from build123d import *

# Parameters (mm, degrees)
F1_DEPTH = 500
F2_DEPTH = 400
F3_T     = -22
F5_DEPTH = 25


# Not quite as in the source:
# - a shell that OpenCascade refuses in one call is made with other operations: the cavity is built on its own and cut out


with BuildPart() as f1:
    # F0 (on Top) → F1 (new body)
    with BuildSketch(Plane.XY):
        Polygon((0, 0), (-1050, 0), (-1050, -22), (-420.8932188135, -22), (-22, -420.8932188135), (-22, -1028), (-500, -1028), (-500, -1050), (0, -1050), align=None)
        Polygon((-389.7805204412, -22), (-22, -22), (-22, -389.7805204412), align=None, mode=Mode.SUBTRACT)
        Polygon((-420.8932188135, -22), (-1050, -22), (-1050, -500), (-650, -500), (-500, -650), (-500, -1028), (-22, -1028), (-22, -420.8932188135), align=None)
    extrude(amount=-F1_DEPTH)

    # F0 (on Top) → F2 (join)
    with BuildSketch(Plane.XY):
        Polygon((0, 0), (-1050, 0), (-1050, -22), (-420.8932188135, -22), (-22, -420.8932188135), (-22, -1028), (-500, -1028), (-500, -1050), (0, -1050), align=None)
        Polygon((-389.7805204412, -22), (-22, -22), (-22, -389.7805204412), align=None, mode=Mode.SUBTRACT)
    extrude(amount=F2_DEPTH)

    # F3: a shell. OpenCascade refuses it in one call, so the cavity is built on its own and cut out:
    # the body offset inwards by the wall thickness, plus a prism from it out through each open face.
    f3_core = offset(f1.part, amount=F3_T, kind=Kind.INTERSECTION, mode=Mode.PRIVATE)
    f3_exits = [f3_core.faces().sort_by_distance(p)[0] for p in [
        (-463.695201, -463.695201, -478),
    ]]
    add(f3_core, mode=Mode.SUBTRACT)
    extrude(f3_exits, amount=-F3_T, mode=Mode.SUBTRACT)

    # F4 (on face) → F5 (cut)
    with BuildSketch(Plane.XZ.offset(1050)):
        with BuildLine():
            ThreePointArc((-500, 248), (-455.4802307404, 355.4802307404), (-348, 400))
            Line((-348, 400), (-500, 400))
            Line((-500, 400), (-500, 248))
        make_face()
    extrude(amount=-F5_DEPTH, mode=Mode.SUBTRACT)


solid = f1.part
Build history of the part. All positions in model axes, mm. A direction names the side the tool comes from. Coordinates: 2 decimals unless noted, no trailing zeros. Order: outer loops, then holes, each group sorted by start corner. A loop starts at its lowest first (then second) coordinate and runs counter-clockwise, first axis right, second up. Notation, with made-up numbers: (55, 14.5) - (95, 14.5) arc R17 cw to (95, 33.5) - close; hole circle Ø8 at (87.5, 6). An arc over 180 degrees is marked (long way). Write each question's results on one line, items separated by ' | '. Start each with the question number.
Item 1: Band-saw the part on A-A on z = -104.5. Write the cut outline in (x, y), and give its area (3 significant figures).
Item 2: Mould opens along X. For faces 1 (the face through (0, -532, -56)), 2 (the face through (-500, -847, -214)), 3 (the face through (-560.584, -558.303, -257.654)), 4 (the face through (-740, -22, 197)) say: released by +X, released by -X, zero draft, split by the parting line, or undercut.
Item 3: Wall check: probe 1 along X at (y, z) = (-684, -312.5); probe 2 along X at (y, z) = (-324, -179). Give the ranges that are in metal, low to high. Write a range as [from, to].
Item 4: Band-saw the part on C-C on y = -343. Write the cut outline in (x, z).
Item 5: Band-saw the part on B-B on x = -149.5. Write the cut outline in (y, z), and give its area (3 significant figures).
Item 6: Band-saw the part on D-D on z = 288. Write the cut outline in (x, y).
Item 7: Flat gauge pins, fed straight in: pin 1 (4 mm diameter, centred on y = -740.5, z = 138, fed in from -X); pin 2 (5 mm diameter, centred on x = -633.5, y = -131.5, fed in from -Z). Where does each tip first touch, or does it go through?
Item 8: Tool access for faces 5 (the face through (-203.32, -208.46, -56.3)), 6 (the face through (-429, -406, 0)), 7 (the face through (-247, -1028, -258)), 8 (the face through (-853, -500, -246)): list every direction of +Z, -Z, +X, -X, +Y, -Y with a clear straight run to the whole face (end or side of a thin tool).
Numbers:
1) outline: (-1050, -500) - (-650, -500) - (-500, -650) - (-500, -1050) - (0, -1050) - (0, 0) - (-1050, 0) - close; hole (-1028, -478) - (-640.89, -478) - (-478, -640.89) - (-478, -1028) - (-22, -1028) - (-22, -420.89) - (-420.89, -22) - (-1028, -22) - close; hole (-389.78, -22) - (-22, -389.78) - (-22, -22) - close | area: 100,000 mm^2
2) face 1: released by +X | face 2: released by -X | face 3: undercut | face 4: zero draft
3) probe 1: [-500, -478], [-22, 0] | probe 2: [-1050, -1028], [-118.89, -87.78], [-22, 0]
4) outline: (-1050, -500) - (-1028, -500) - (-1028, -22) - (-99.89, -22) - (-99.89, -500) - (-68.78, -500) - (-68.78, 400) - (-99.89, 400) - (-99.89, 0) - (-1050, 0) - close; (-22, -500) - (0, -500) - (0, 400) - (-22, 400) - close
5) outline: (-1050, -500) - (-1028, -500) - (-1028, -22) - (-293.39, -22) - (-293.39, -500) - (-262.28, -500) - (-262.28, 400) - (-293.39, 400) - (-293.39, 0) - (-1028, 0) - (-1028, 400) - (-1050, 400) - close; (-22, -500) - (0, -500) - (0, 400) - (-22, 400) - close | area: 83,800 mm^2
6) outline: (-1050, -22) - (-420.89, -22) - (-22, -420.89) - (-22, -1028) - (-494.64, -1028) - (-494.64, -1050) - (0, -1050) - (0, 0) - (-1050, 0) - close; hole (-389.78, -22) - (-22, -389.78) - (-22, -22) - close
7) pin 1: x = -22 | pin 2: z = -22
8) face 5: +Z, -Z | face 6: +Z, -X | face 7: -Z | face 8: +Z, -Z, -X, -Y
